The model under review builds one solid part; all positions refer to its coordinate system, in mm. Face numbers are marked on the shaded views. A direction names the side the tool comes from. Coordinates: 2 decimals unless noted, no trailing zeros. Loops run counter-clockwise (first coordinate to the right, second up) from the corner with the lowest first, then second, coordinate; pieces in that order, holes last. Notation, with made-up numbers: M 36,-7.5 L 49,-7.5 A18 ccw 49,11.5 Z; hole C 24.5,19 d2. An arc over 180 degrees is marked long. Use CSV: the item, a comma, the result in double quotes. Start each with the question number.
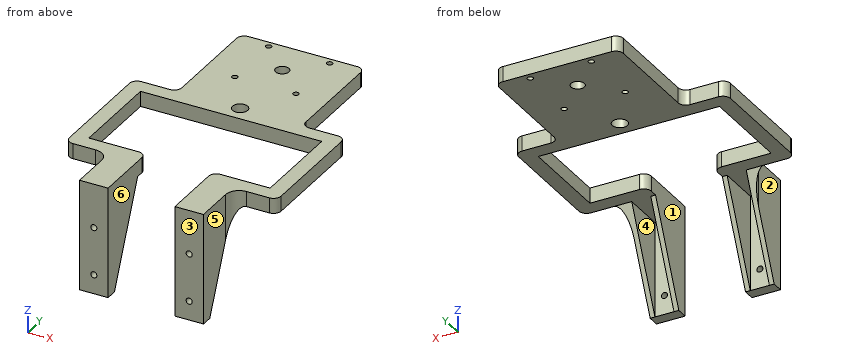
from build123d import *

# Parameters (mm, degrees)
SKETCH_R     = 4
SKETCH_R_2   = 3.5
SKETCH_R_3   = 1.5
PAD_DEPTH    = 8
SKETCH001_W  = 15
SKETCH001_H  = 6
PAD001_DEPTH = 50
PAD002_DEPTH = 2.5
PAD003_DEPTH = 2.5
PAD004_DEPTH = 2.5
PAD005_DEPTH = 2.5
SKETCH006_R  = 1.6
POCKET_DEPTH = 6
FILLET_R     = 7
FILLET001_R  = 4
FILLET002_R  = 4


with BuildPart() as part:
    # Sketch → Pad (new body)
    with BuildSketch(Plane.XY):
        Polygon((-17.5, 0), (-32.5, 0), (-32.5, 28), (-55.5, 28), (-55.5, 93), (-32.5, 93), (-32.5, 153), (32.5, 153), (32.5, 93), (55.5, 93), (55.5, 28), (32.5, 28), (32.5, 0), (17.5, 0), (17.5, 36), (47.5, 36), (47.5, 85), (17.5, 85), (-17.5, 85), (-47.5, 85), (-47.5, 36), (-17.5, 36), align=None)
        with Locations((0, 93.5)):
            Circle(SKETCH_R, mode=Mode.SUBTRACT)
        with Locations((0, 133.5)):
            Circle(SKETCH_R_2, mode=Mode.SUBTRACT)
        with Locations((-16, 149.5)):
            Circle(SKETCH_R_3, mode=Mode.SUBTRACT)
        with Locations((16, 149.5)):
            Circle(SKETCH_R_3, mode=Mode.SUBTRACT)
        with Locations((16, 117.5)):
            Circle(SKETCH_R_3, mode=Mode.SUBTRACT)
        with Locations((-16, 117.5)):
            Circle(SKETCH_R_3, mode=Mode.SUBTRACT)
    extrude(amount=PAD_DEPTH)

    # Sketch001 (on Face20 of Pad) → Pad001 (join)
    with BuildSketch(Plane(origin=(0, 0, 0), x_dir=(1, 0, 0), z_dir=(0, 0, -1))):
        with Locations((-25, -3)):
            Rectangle(SKETCH001_W, SKETCH001_H)
        with Locations((25, -3)):
            Rectangle(SKETCH001_W, SKETCH001_H)
    extrude(amount=PAD001_DEPTH)

    # Sketch002 (on Face31 of Pad001) → Pad002 (join)
    with BuildSketch(Plane.YZ.offset(32.5)):
        Polygon((6, 0), (6, -50), (28, 0), align=None)
    extrude(amount=-PAD002_DEPTH)

    # Sketch003 (on Face14 of Pad002) → Pad003 (join)
    with BuildSketch(Plane(origin=(17.5, 0, 0), x_dir=(0, -1, 0), z_dir=(-1, 0, 0))):
        Polygon((-6, 0), (-28, 0), (-6, -50), align=None)
    extrude(amount=-PAD003_DEPTH)

    # Sketch004 (on Face3 of Pad003) → Pad004 (join)
    with BuildSketch(Plane(origin=(-32.5, 0, 0), x_dir=(0, -1, 0), z_dir=(-1, 0, 0))):
        Polygon((-6, -50), (-6, 0), (-28, 0), align=None)
    extrude(amount=-PAD004_DEPTH)

    # Sketch005 (on Face20 of Pad004) → Pad005 (join)
    with BuildSketch(Plane.YZ.offset(-17.5)):
        Polygon((28, 0), (6, 0), (6, -50), align=None)
    extrude(amount=-PAD005_DEPTH)

    # Sketch006 (on Face2 of Pad005) → Pocket (cut)
    with BuildSketch(Plane.XZ):
        with Locations((25, -40)):
            Circle(SKETCH006_R)
        with Locations((25, -15)):
            Circle(SKETCH006_R)
        with Locations((-25, -15)):
            Circle(SKETCH006_R)
        with Locations((-25, -40)):
            Circle(SKETCH006_R)
    extrude(amount=-POCKET_DEPTH, mode=Mode.SUBTRACT)

    # Fillet
    fillet_edges = [part.edges().sort_by_distance(p)[0] for p in [
        (-32.5, 28, 4),
        (32.5, 28, 4),
    ]]
    fillet(fillet_edges, radius=FILLET_R)

    # Fillet001
    fillet001_edges = [part.edges().sort_by_distance(p)[0] for p in [
        (-55.5, 28, 4),
        (-55.5, 93, 4),
        (-32.5, 93, 4),
        (-32.5, 153, 4),
        (32.5, 153, 4),
        (32.5, 93, 4),
        (55.5, 93, 4),
        (55.5, 28, 4),
    ]]
    fillet(fillet001_edges, radius=FILLET001_R)

    # Fillet002
    fillet002_edges = [part.edges().sort_by_distance(p)[0] for p in [
        (17.5, 36, 4),
        (-17.5, 36, 4),
    ]]
    fillet(fillet002_edges, radius=FILLET002_R)


solid = part.part
1. Add section D-D (z = -20.5). Write out the cut boundary in (x, y).
2. Add section C-C (x = 42). Write out the cut boundary in (y, z), plus the area to 3 significant figures.
3. Add section B-B (y = 133.5). Write out the cut boundary in (x, z).
4. Insertion check: pin 1 Ø10.5 at (y, z) = (6, -7.5) entering from -X; pin 2 Ø2.5 at (x, y) = (16, 149.5) entering from +Z; pin 3 Ø8 at (x, z) = (-25, -14) entering from +Y; pin 4 Ø23 at (y, z) = (6, -31) entering from +X. Each pin has a flat end and moves straight along its axis. Give the tip position at first contact, or say it passes through.
5. To check wall thickness, follow line 1 along X through (y, z) = (9, -10); line 2 along Z through (x, y) = (-25, 2.65); line 3 along Y through (x, z) = (0, 2.25). State the ranges of each line that lie inside material, in increasing order.
6. For the marked faces 4, 5 and 6, list the 3-axis set-ups (+Z, -Z, +X, -X, +Y, -Y) from which the entire face can be reached by the end or side of a thin tool; tool diameter is ignored.
7. Draft analysis for pull direction X (two halves, no side actions). For the marked faces 1, 2 and 3, state which applies: released by +X, released by -X, zero draft, split by the parting line, or undercut.
8. Add section A-A (z = -40). Write out the cut boundary in (x, y).
Solved:
1,outline,"M -32.5,0 L -17.5,0 L -17.5,18.98 L -20,18.98 L -20,6 L -30,6 L -30,18.98 L -32.5,18.98 Z; M 17.5,0 L 32.5,0 L 32.5,18.98 L 30,18.98 L 30,6 L 20,6 L 20,18.98 L 17.5,18.98 Z"
2,outline,"M 28,0 L 36,0 L 36,8 L 28,8 Z; M 85,0 L 93,0 L 93,8 L 85,8 Z"
2,area,"128 mm^2"
3,outline,"M -32.5,0 L -3.5,0 L -3.5,8 L -32.5,8 Z; M 3.5,0 L 32.5,0 L 32.5,8 L 3.5,8 Z"
4,pin 1,"stops at x = -32.5"
4,pin 2,"passes through"
4,pin 3,"stops at y = 6"
4,pin 4,"stops at x = 32.5"
5,line 1,"x = -32.5 to -30, -20 to -17.5, 17.5 to 20, 30 to 32.5"
5,line 2,"z = -50 to -41.6, -38.4 to -16.6, -13.4 to 8"
5,line 3,"y = 85 to 89.5, 97.5 to 130, 137 to 153"
6,face 4,"-Z, +Y"
6,face 5,"+Z, -Z, +X, -Y"
6,face 6,"+Z, -Z, -Y"
7,face 1,"undercut"
7,face 2,"released by -X"
7,face 3,"zero draft"
8,outline,"M -32.5,0 L -26.6,0 L -26.6,6 L -30,6 L -30,10.4 L -32.5,10.4 Z; M -23.4,0 L -17.5,0 L -17.5,10.4 L -20,10.4 L -20,6 L -23.4,6 Z; M 17.5,0 L 23.4,0 L 23.4,6 L 20,6 L 20,10.4 L 17.5,10.4 Z; M 26.6,0 L 32.5,0 L 32.5,10.4 L 30,10.4 L 30,6 L 26.6,6 Z"
